from build123d import *

# Parameters (mm, degrees)
SKETCH1_W                       = 63
SKETCH1_H                       = 44
BOSS_EXTRUDE1_DEPTH             = 1.5
BOSS_EXTRUDE2_DEPTH             = 3
SKETCH2_R                       = 11.375
SKETCH2_R_2                     = 1.5
SKETCH2_R_3                     = 2.05
CUT_EXTRUDE1_DEPTH              = 96.44762962
FILLET1_R                       = 4
TAP_DRILL_FOR_M3X0_5_TAP1_D     = 2.5
TAP_DRILL_FOR_M3X0_5_TAP1_DEPTH = 4
TAP_DRILL_FOR_M3X0_5_TAP1_TIP   = 0.751075774
FILLET2_R                       = 2


with BuildPart() as part:
    # Sketch1 → Boss-Extrude1 (new, symmetric)
    with BuildSketch(Plane.XY):
        Rectangle(SKETCH1_W, SKETCH1_H)
    extrude(amount=BOSS_EXTRUDE1_DEPTH, both=True)

    # Sketch3 → Boss-Extrude2 (add)
    with BuildSketch(Plane.XY.offset(1.5)):
        Polygon((31.5, -12), (91.5, -12), (91.5, 27), (51.5, 27), (51.5, 22), (31.5, 22), align=None)
    extrude(amount=-BOSS_EXTRUDE2_DEPTH)

    # Sketch2 → Cut-Extrude1 (cut, through all)
    with BuildSketch(Plane.XY.offset(1.5)):
        with Locations((9.5, 0)):
            Circle(SKETCH2_R)
        with Locations((-6, 15.5)):
            Circle(SKETCH2_R_2)
        with Locations((25, 15.5)):
            Circle(SKETCH2_R_2)
        with Locations((25, -15.5)):
            Circle(SKETCH2_R_2)
        with Locations((-6, -15.5)):
            Circle(SKETCH2_R_2)
        with Locations((-21.5, 15)):
            Circle(SKETCH2_R_3)
        with Locations((-21.5, -15)):
            Circle(SKETCH2_R_3)
    extrude(amount=-CUT_EXTRUDE1_DEPTH, mode=Mode.SUBTRACT)

    # Fillet1
    fillet1_edges = [part.edges().sort_by_distance(p)[0] for p in [
        (31.5, -22, 0),
        (-31.5, -22, 0),
        (-31.5, 22, 0),
    ]]
    fillet(fillet1_edges, radius=FILLET1_R)

    # Tap Drill for M3x0.5 Tap1
    with Locations(Plane.XY.offset(1.5)):
        with Locations((57.5, 21), (85.5, 21), (85.5, 5), (57.5, 5)):
            Hole(TAP_DRILL_FOR_M3X0_5_TAP1_D / 2, depth=TAP_DRILL_FOR_M3X0_5_TAP1_DEPTH)
            with Locations((0, 0, -(TAP_DRILL_FOR_M3X0_5_TAP1_DEPTH + TAP_DRILL_FOR_M3X0_5_TAP1_TIP / 2))):  # 118° drill point
                Cone(0, TAP_DRILL_FOR_M3X0_5_TAP1_D / 2, TAP_DRILL_FOR_M3X0_5_TAP1_TIP, mode=Mode.SUBTRACT)

    # Fillet2
    fillet2_edges = [part.edges().sort_by_distance(p)[0] for p in [
        (31.5, -12, 0),
        (51.5, 22, 0),
        (51.5, 27, 0),
        (91.5, 27, 0),
        (91.5, -12, 0),
    ]]
    fillet(fillet2_edges, radius=FILLET2_R)


solid = part.part
Design review of the part built by this model. Coordinates are the model's own, in mm. A direction names the side the tool comes from. Coordinates: 2 decimals unless noted, no trailing zeros. Order: outer loops, then holes, each group sorted by start corner. A loop starts at its lowest first (then second) coordinate and runs counter-clockwise, first axis right, second up. Notation, with made-up numbers: (68.25, -2.75) -> (100.25, -2.75) arc R23 ccw to (100.25, 7.25) -> close; hole circle Ø6 at (65.5, 19). An arc over 180 degrees is marked (long way). Use one line per item in the form item = value. Start each with the question number.
(1) The part is to be moulded in two halves that separate along X. For faces 4 (the cylindrical face through (52.1, 26.43, -0.02)), 5 (the cylindrical face through (30.359, -20.797, 0.021)), 6 (the cylindrical face through (-21.944, 12.999, 0.021)), say which applies: +X half, -X half, draft (parallel to the pull), parting line (faces both ways), or undercut.
(2) Insertion check: pin 1 (1.5 mm diameter, centred on y = -17, z = 0, fed in from +X); pin 2 (0.8 mm diameter, centred on y = 24.5, z = 0.5, fed in from -X); pin 3 (1 mm diameter, centred on x = 43, z = 1, fed in from +Y). Each pin has a flat end and moves straight along its axis. Give the tip position at first contact, or say it passes through.
(3) For probe 1 along Y at (x, z) = (25, -0.25); probe 2 along Y at (x, z) = (-21.5, -0.25); probe 3 along Y at (x, z) = (54, 0.5), list the stretches that pass through material, from the lowest coordinate up.
(4) Add section A-A on z = -0.3. Give the number of separate pieces and of enclosed holes in the cut face, plus the area to 3 significant figures.
(5) Add section D-D on x = 11.5. State the section outline as (y, z) points, plus the area to 3 significant figures.
(6) For faces 1 (the flat face through (12, 22, 0)), 2 (the flat face through (31.5, -16, 0)), 3 (the cylindrical face through (23.5, -15.43, 0.02)), list the 3-axis set-ups (+Z, -Z, +X, -X, +Y, -Y) from which the entire face can be reached by the end or side of a thin tool; tool diameter is ignored.
(7) Add section B-B on x = 57.5. State the section outline as (y, z) points.
(8) Add section C-C on y = 5. State the section outline as (x, z) points, plus the area to 3 significant figures.
Answer block:
q1.face_4 = -X half
q1.face_5 = +X half
q1.face_6 = undercut
q2.pin_1 = 31.5
q2.pin_2 = 51.5
q2.pin_3 = 22
q3.probe_1 = -22 to -17, -14 to 14, 17 to 22
q3.probe_2 = -22 to -17.05, -12.95 to 12.95, 17.05 to 22
q3.probe_3 = -12 to 27
q4.separate_pieces = 1
q4.enclosed_holes = 11
q4.area = 4,520 mm²
q5.outline = (-22, -1.5) -> (-11.2, -1.5) -> (-11.2, 1.5) -> (-22, 1.5) -> close; (11.2, -1.5) -> (22, -1.5) -> (22, 1.5) -> (11.2, 1.5) -> close
q5.area = 64.8 mm²
q6.face_1 = +Z, -Z, -X, +Y
q6.face_2 = +Z, -Z, +X, -Y
q6.face_3 = +Z, -Z
q7.outline = (-12, -1.5) -> (3.75, -1.5) -> (3.75, 1.5) -> (-12, 1.5) -> close; (6.25, -1.5) -> (19.75, -1.5) -> (19.75, 1.5) -> (6.25, 1.5) -> close; (22.25, -1.5) -> (27, -1.5) -> (27, 1.5) -> (22.25, 1.5) -> close
q8.outline = (-31.5, -1.5) -> (-0.72, -1.5) -> (-0.72, 1.5) -> (-31.5, 1.5) -> close; (19.72, -1.5) -> (56.25, -1.5) -> (56.25, 1.5) -> (19.72, 1.5) -> close; (58.75, -1.5) -> (84.25, -1.5) -> (84.25, 1.5) -> (58.75, 1.5) -> close; (86.75, -1.5) -> (91.5, -1.5) -> (91.5, 1.5) -> (86.75, 1.5) -> close
q8.area = 293 mm²
